Here's the drawing with two shaded views (mm, measured from the low corner). I have some questions. A direction names the side the tool comes from. Give positions to 0.01 mm unless a question says otherwise; leave off trailing zeros. Loops run counter-clockwise (first coordinate to the right, second up) from the corner with the lowest first, then second, coordinate; pieces in that order, holes last. Notation, with made-up numbers: (41.5, 85.25) - (98.5, 85.25) arc R17 cw to (98.5, 99.25) - close; hole circle Ø8 at (88.25, -30.75). An arc over 180 degrees is marked (long way). Answer as a JSON object with one key per item and string values. Group by question number.
Item 1: Suppose I cut it at C-C on x = 87.1. Write out the boundary of the cut face in (y, z).
Item 2: Thinking about a two-plate mould opening in Z: for the marked faces 1, 2 and 3, which applies, pulls with the +Z half, pulls with the -Z half, needs draft (parallel to the pull), parting line crosses it, or undercut?
Item 3: Please list where these lines run through material, in increasing order: L1, parallel to X at y = 0.9, z = 8.9; L2, parallel to Z at x = 11, y = 12.25; L3, parallel to X at y = 14.5, z = 50 (1 decimal).
Item 4: Suppose I cut it at B-B on y = 12.5. Write out the boundary of the cut face in (x, z) (1 decimal), and give its area (3 significant figures).
Item 5: Suppose I cut it at A-A on z = 8.9. Write out the boundary of the cut face in (x, y).
Item 6: Suppose I cut it at D-D on x = 38. Write out the boundary of the cut face in (y, z), and give its area (3 significant figures).
Item 7: Which directions (+Z, -Z, +X, -X, +Y, -Y) give clear straight access to the entire face, cutting with the end or side of a thin tool? Please do the marked faces 4, 5, 6, 7 and 8.
Item 8: Will these pins go through, and if not, where does the flat tip stop? pin 1 (3 mm diameter, centred on x = 34, y = 16, fed in from +Z); pin 2 (1 mm diameter, centred on x = 48, z = 9.5, fed in from +Y); pin 3 (6 mm diameter, centred on y = 8.5, z = 57, fed in from -X); pin 4 (1.5 mm diameter, centred on y = 5.5, z = 13.5, fed in from -X).
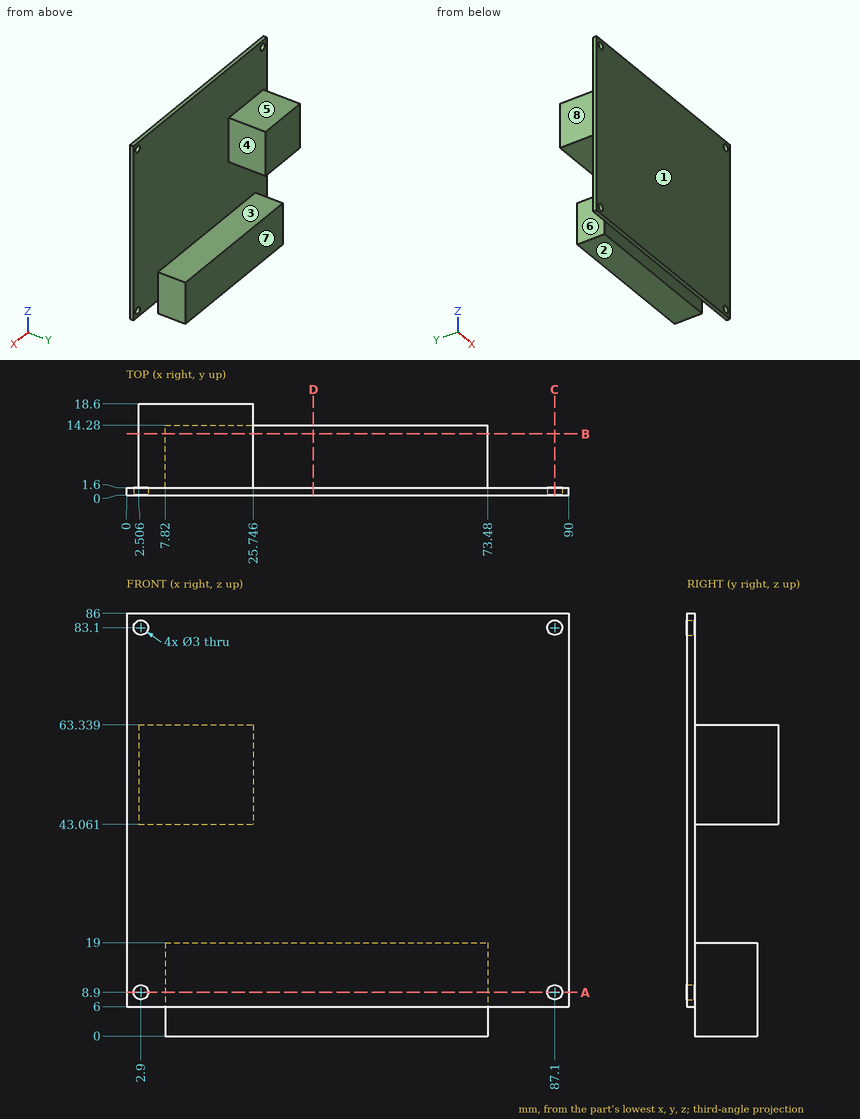
Worked out:
{
 "1": {"outline": "(0, 6) - (1.6, 6) - (1.6, 7.4) - (0, 7.4) - close; (0, 10.4) - (1.6, 10.4) - (1.6, 81.6) - (0, 81.6) - close; (0, 84.6) - (1.6, 84.6) - (1.6, 86) - (0, 86) - close"},
 "2": {"face 1": "needs draft", "face 2": "pulls with the -Z half", "face 3": "undercut"},
 "3": {"L1": "x = 0 to 1.4, 4.4 to 85.6, 88.6 to 90", "L2": "z = 0 to 19, 43.06 to 63.34", "L3": "x = 2.5 to 25.7"},
 "4": {"outline": "(2.5, 43.1) - (25.7, 43.1) - (25.7, 63.3) - (2.5, 63.3) - close; (7.8, 0) - (73.5, 0) - (73.5, 19) - (7.8, 19) - close", "area": "1,720 mm2"},
 "5": {"outline": "(0, 0) - (1.4, 0) - (1.4, 1.6) - (0, 1.6) - close; (4.4, 0) - (85.6, 0) - (85.6, 1.6) - (73.48, 1.6) - (73.48, 14.28) - (7.82, 14.28) - (7.82, 1.6) - (4.4, 1.6) - close; (88.6, 0) - (90, 0) - (90, 1.6) - (88.6, 1.6) - close"},
 "6": {"outline": "(0, 6) - (1.6, 6) - (1.6, 0) - (14.28, 0) - (14.28, 19) - (1.6, 19) - (1.6, 86) - (0, 86) - close", "area": "369 mm2"},
 "7": {"face 4": "+Z, +X, +Y", "face 5": "+Z, +X, -X, +Y", "face 6": "-Z, -X, +Y", "face 7": "-Z, +X, -X, +Y", "face 8": "+Z, -Z, -X, +Y"},
 "8": {"pin 1": "passes through", "pin 2": "stops at y = 14.28", "pin 3": "stops at x = 2.51", "pin 4": "stops at x = 7.82"}
}
